The model under review builds one solid part; all positions refer to its coordinate system, in mm. A direction names the side the tool comes from. Coordinates: 2 decimals unless noted, no trailing zeros. Write each loop counter-clockwise with the first axis right and the second up, starting at its lowest first coordinate (ties: lowest second). Pieces come first, ordered by that corner, then holes. Notation, with made-up numbers: (51.5, 58.25) - (58.5, 58.25) arc R22 ccw to (58.5, 80.25) - close; hole circle Ø10 at (3, 83.25). An arc over 180 degrees is marked (long way). Use one line per item in the form item = value. Start each with the question number.
```python
from build123d import *

# Parameters (mm, degrees)
SKETCH1_W             = 18.7
SKETCH1_H             = 6.4
BOSS_EXTRUDE1_DEPTH   = 13
SKETCH2_W             = 13
SKETCH2_H             = 0.7
SKETCH2_W_2           = 0.5
SKETCH2_H_2           = 6.4
SKETCH2_W_3           = 1
BOSS_EXTRUDE2_DEPTH   = 2
CUT_EXTRUDE1_REACH    = 17
SKETCH3_R             = 0.9
CUT_EXTRUDE2_REACH    = 8.4
SKETCH5_R             = 1.1
CUT_EXTRUDE3_DEPTH    = 5.4
SKETCH6_R             = 1.1
CUT_EXTRUDE4_DEPTH    = 6.3
SKETCH7_R             = 1.1
CUT_EXTRUDE5_DEPTH    = 7
SKETCH8_R             = 1.1
CUT_EXTRUDE6_DEPTH    = 7.8
SKETCH10_W            = 6.4
SKETCH10_H            = 1
BOSS_EXTRUDE3_DEPTH   = 0.5
SKETCH11_W            = 6.4
SKETCH11_H            = 1
BOSS_EXTRUDE4_DEPTH   = 0.5
CHAMFER1_SIZE         = 0.5
CHAMFER1_SIZE2        = 0.3
CHAMFER1_PART_2_SIZE  = 0.5
CHAMFER1_PART_2_SIZE2 = 0.3


with BuildPart() as part:
    # Sketch1 → Boss-Extrude1 (new body)
    with BuildSketch(Plane(origin=(0, 0, 0), x_dir=(1, 0, 0), z_dir=(0, 1, 0))):
        Rectangle(SKETCH1_W, SKETCH1_H)
    extrude(amount=BOSS_EXTRUDE1_DEPTH)

    # Sketch2 → Boss-Extrude2 (add)
    with BuildSketch(Plane.XZ):
        with Locations((0.15, 2.85)):
            Rectangle(SKETCH2_W, SKETCH2_H)
        with Locations((0.15, -2.85)):
            Rectangle(SKETCH2_W, SKETCH2_H)
        with Locations((-9.1, 0)):
            Rectangle(SKETCH2_W_2, SKETCH2_H_2)
        with Locations((8.85, 0)):
            Rectangle(SKETCH2_W_3, SKETCH2_H_2)
    extrude(amount=BOSS_EXTRUDE2_DEPTH)

    # Sketch3 → Cut-Extrude1 (cut, up to next)
    with BuildSketch(Plane(origin=(0, 13, 0), x_dir=(1, 0, 0), z_dir=(0, 1, 0)), mode=Mode.PRIVATE) as cut_extrude1_sk1:
        with Locations(Location((4.25, -1.25, 0), (0, 0, 270))):  # turned: the seam where the file's is
            Circle(SKETCH3_R)
    cut_extrude1_tool1 = extrude(cut_extrude1_sk1.sketch, amount=-CUT_EXTRUDE1_REACH, mode=Mode.PRIVATE) & part.part
    add(cut_extrude1_tool1.solids().sort_by_distance((4.25, 13, 1.25))[0], mode=Mode.SUBTRACT)
    # Sketch3 → Cut-Extrude1 (cut, up to next)
    with BuildSketch(Plane(origin=(0, 13, 0), x_dir=(1, 0, 0), z_dir=(0, 1, 0)), mode=Mode.PRIVATE) as cut_extrude1_sk2:
        with Locations(Location((1.75, -1.25, 0), (0, 0, 270))):  # turned: the seam where the file's is
            Circle(SKETCH3_R)
    cut_extrude1_tool2 = extrude(cut_extrude1_sk2.sketch, amount=-CUT_EXTRUDE1_REACH, mode=Mode.PRIVATE) & part.part
    add(cut_extrude1_tool2.solids().sort_by_distance((1.75, 13, 1.25))[0], mode=Mode.SUBTRACT)
    # Sketch3 → Cut-Extrude1 (cut, up to next)
    with BuildSketch(Plane(origin=(0, 13, 0), x_dir=(1, 0, 0), z_dir=(0, 1, 0)), mode=Mode.PRIVATE) as cut_extrude1_sk3:
        with Locations(Location((-0.75, -1.25, 0), (0, 0, 270))):  # turned: the seam where the file's is
            Circle(SKETCH3_R)
    cut_extrude1_tool3 = extrude(cut_extrude1_sk3.sketch, amount=-CUT_EXTRUDE1_REACH, mode=Mode.PRIVATE) & part.part
    add(cut_extrude1_tool3.solids().sort_by_distance((-0.75, 13, 1.25))[0], mode=Mode.SUBTRACT)
    # Sketch3 → Cut-Extrude1 (cut, up to next)
    with BuildSketch(Plane(origin=(0, 13, 0), x_dir=(1, 0, 0), z_dir=(0, 1, 0)), mode=Mode.PRIVATE) as cut_extrude1_sk4:
        with Locations(Location((-3.25, -1.25, 0), (0, 0, 270))):  # turned: the seam where the file's is
            Circle(SKETCH3_R)
    cut_extrude1_tool4 = extrude(cut_extrude1_sk4.sketch, amount=-CUT_EXTRUDE1_REACH, mode=Mode.PRIVATE) & part.part
    add(cut_extrude1_tool4.solids().sort_by_distance((-3.25, 13, 1.25))[0], mode=Mode.SUBTRACT)
    # Sketch3 → Cut-Extrude1 (cut, up to next)
    with BuildSketch(Plane(origin=(0, 13, 0), x_dir=(1, 0, 0), z_dir=(0, 1, 0)), mode=Mode.PRIVATE) as cut_extrude1_sk5:
        with Locations(Location((4.25, 1.25, 0), (0, 0, 270))):  # turned: the seam where the file's is
            Circle(SKETCH3_R)
    cut_extrude1_tool5 = extrude(cut_extrude1_sk5.sketch, amount=-CUT_EXTRUDE1_REACH, mode=Mode.PRIVATE) & part.part
    add(cut_extrude1_tool5.solids().sort_by_distance((4.25, 13, -1.25))[0], mode=Mode.SUBTRACT)
    # Sketch3 → Cut-Extrude1 (cut, up to next)
    with BuildSketch(Plane(origin=(0, 13, 0), x_dir=(1, 0, 0), z_dir=(0, 1, 0)), mode=Mode.PRIVATE) as cut_extrude1_sk6:
        with Locations(Location((1.75, 1.25, 0), (0, 0, 270))):  # turned: the seam where the file's is
            Circle(SKETCH3_R)
    cut_extrude1_tool6 = extrude(cut_extrude1_sk6.sketch, amount=-CUT_EXTRUDE1_REACH, mode=Mode.PRIVATE) & part.part
    add(cut_extrude1_tool6.solids().sort_by_distance((1.75, 13, -1.25))[0], mode=Mode.SUBTRACT)
    # Sketch3 → Cut-Extrude1 (cut, up to next)
    with BuildSketch(Plane(origin=(0, 13, 0), x_dir=(1, 0, 0), z_dir=(0, 1, 0)), mode=Mode.PRIVATE) as cut_extrude1_sk7:
        with Locations(Location((-0.75, 1.25, 0), (0, 0, 270))):  # turned: the seam where the file's is
            Circle(SKETCH3_R)
    cut_extrude1_tool7 = extrude(cut_extrude1_sk7.sketch, amount=-CUT_EXTRUDE1_REACH, mode=Mode.PRIVATE) & part.part
    add(cut_extrude1_tool7.solids().sort_by_distance((-0.75, 13, -1.25))[0], mode=Mode.SUBTRACT)
    # Sketch3 → Cut-Extrude1 (cut, up to next)
    with BuildSketch(Plane(origin=(0, 13, 0), x_dir=(1, 0, 0), z_dir=(0, 1, 0)), mode=Mode.PRIVATE) as cut_extrude1_sk8:
        with Locations(Location((-3.25, 1.25, 0), (0, 0, 270))):  # turned: the seam where the file's is
            Circle(SKETCH3_R)
    cut_extrude1_tool8 = extrude(cut_extrude1_sk8.sketch, amount=-CUT_EXTRUDE1_REACH, mode=Mode.PRIVATE) & part.part
    add(cut_extrude1_tool8.solids().sort_by_distance((-3.25, 13, -1.25))[0], mode=Mode.SUBTRACT)

    # Sketch4 → Cut-Extrude2 (cut, up to next)
    with BuildSketch(Plane(origin=(0, 0, -3.2), x_dir=(-1, 0, 0), z_dir=(0, 0, -1)), mode=Mode.PRIVATE) as cut_extrude2_sk1:
        with BuildLine():
            Line((-9.35, 13), (9.35, 13))
            Line((9.35, 13), (9.35, 9.790050428))
            add(Edge.make_bspline(
                [(9.35, 9.790050428), (-0.455442008, 7.925691322), (-9.35, 3.892093752)],
                knots=[1.786761572, 1.786761572, 1.786761572, 2.052876958, 2.052876958, 2.052876958], degree=2, weights=[1, 0.991160878, 1]))
            Line((-9.35, 3.892093752), (-9.35, 13))
        make_face()
    cut_extrude2_tool1 = extrude(cut_extrude2_sk1.sketch, amount=-CUT_EXTRUDE2_REACH, mode=Mode.PRIVATE) & part.part
    add(cut_extrude2_tool1.solids().sort_by_distance((1.591729, 9.871634, -3.2))[0], mode=Mode.SUBTRACT)

    # Sketch5 → Cut-Extrude3 (cut)
    with BuildSketch(Plane.XZ):
        with Locations(Location((4.25, -1.25, 0), (0, 0, 270))):  # turned: the seam where the file's is
            Circle(SKETCH5_R)
        with Locations(Location((4.25, 1.25, 0), (0, 0, 270))):  # turned: the seam where the file's is
            Circle(SKETCH5_R)
    extrude(amount=-CUT_EXTRUDE3_DEPTH, mode=Mode.SUBTRACT)

    # Sketch6 → Cut-Extrude4 (cut)
    with BuildSketch(Plane.XZ):
        with Locations(Location((1.75, 1.25, 0), (0, 0, 270))):  # turned: the seam where the file's is
            Circle(SKETCH6_R)
        with Locations(Location((1.75, -1.25, 0), (0, 0, 270))):  # turned: the seam where the file's is
            Circle(SKETCH6_R)
    extrude(amount=-CUT_EXTRUDE4_DEPTH, mode=Mode.SUBTRACT)

    # Sketch7 → Cut-Extrude5 (cut)
    with BuildSketch(Plane.XZ):
        with Locations(Location((-0.75, 1.25, 0), (0, 0, 270))):  # turned: the seam where the file's is
            Circle(SKETCH7_R)
        with Locations(Location((-0.75, -1.25, 0), (0, 0, 270))):  # turned: the seam where the file's is
            Circle(SKETCH7_R)
    extrude(amount=-CUT_EXTRUDE5_DEPTH, mode=Mode.SUBTRACT)

    # Sketch8 → Cut-Extrude6 (cut)
    with BuildSketch(Plane.XZ):
        with Locations(Location((-3.25, 1.25, 0), (0, 0, 270))):  # turned: the seam where the file's is
            Circle(SKETCH8_R)
        with Locations(Location((-3.25, -1.25, 0), (0, 0, 270))):  # turned: the seam where the file's is
            Circle(SKETCH8_R)
    extrude(amount=-CUT_EXTRUDE6_DEPTH, mode=Mode.SUBTRACT)

    # Sketch10 → Boss-Extrude3 (add)
    with BuildSketch(Plane.ZY.offset(-8.35)):
        with Locations((0, -1.5)):
            Rectangle(SKETCH10_W, SKETCH10_H)
    extrude(amount=BOSS_EXTRUDE3_DEPTH)

    # Sketch11 → Boss-Extrude4 (add)
    with BuildSketch(Plane(origin=(-8.85, 0, 0), x_dir=(0, 0, -1), z_dir=(1, 0, 0))):
        with Locations((0, -1.5)):
            Rectangle(SKETCH11_W, SKETCH11_H)
    extrude(amount=BOSS_EXTRUDE4_DEPTH)

    # Chamfer1
    chamfer1_edges = [part.edges().sort_by_distance(p)[0] for p in [
        (7.85, -2, 0),
    ]]
    chamfer1_side = [part.faces().sort_by_distance(p)[0] for p in [
        (8.6, -2, 0),
    ]]
    chamfer(chamfer1_edges, length=CHAMFER1_SIZE, length2=CHAMFER1_SIZE2, reference=chamfer1_side[0])

    # Chamfer1 part 2
    chamfer1_part_2_edges = [part.edges().sort_by_distance(p)[0] for p in [
        (-8.35, -2, 0),
    ]]
    chamfer1_part_2_side = [part.faces().sort_by_distance(p)[0] for p in [
        (-8.85, -2, 0),
    ]]
    chamfer(chamfer1_part_2_edges, length=CHAMFER1_PART_2_SIZE, length2=CHAMFER1_PART_2_SIZE2, reference=chamfer1_part_2_side[0])


solid = part.part
```
1. For faces 3 (the cylindrical face through (-4.129, 8.129, 1.055)), 4 (the cylindrical face through (4.993, 2.662, -0.439)), list the 3-axis set-ups (+Z, -Z, +X, -X, +Y, -Y) from which the entire face can be reached by the end or side of a thin tool; tool diameter is ignored.
2. Take a section at A-A (y = -0.5). State the section outline as (x, z) points, plus the area to 3 significant figures.
3. Take a section at B-B (z = -1.25). Count the separate pieces of the cut face and the enclosed holes in it, plus the area to 3 significant figures.
4. The part is to be moulded in two halves that separate along Z. For faces 1 (the flat face through (-8.85, -0.5, 0)), 2 (the cylindrical face through (3.371, 5.767, 1.055)), say which applies: released by +Z, released by -Z, zero draft, split by the parting line, or undercut.
5. For L1, parallel to Z at x = -3.25, y = 8.1; L2, parallel to X at y = 3.25, z = 1.25; L3, parallel to Z at x = -3.75, y = 5.5, list the stretches that pass through material, from the lowest coordinate up.
6. For P1, Ø1.1, axis at x = 1.75, z = -1.25, coming from the +Y side; P2, Ø2, axis at x = 4.25, z = 1.25, coming from the -Y side; P3, Ø0.6, axis at x = -8.5, z = 0, coming from the +Y side; P4, Ø3, axis at x = -3, z = -0.5, coming from the +Y side, all flat-tipped, find the tip position at first contact; note any pin that passes through.
Returned:
q1.face_3 = +Y, -Y
q1.face_4 = -Y
q2.outline = (-9.35, -3.2) - (-8.85, -3.2) - (-8.85, 3.2) - (-9.35, 3.2) - close; (-6.35, -3.2) - (6.65, -3.2) - (6.65, -2.5) - (-6.35, -2.5) - close; (-6.35, 2.5) - (6.65, 2.5) - (6.65, 3.2) - (-6.35, 3.2) - close; (8.35, -3.2) - (9.35, -3.2) - (9.35, 3.2) - (8.35, 3.2) - close
q2.area = 27.8 mm²
q3.separate_pieces = 5
q3.enclosed_holes = 0
q3.area = 76.7 mm²
q4.face_1 = zero draft
q4.face_2 = undercut
q5.L1 = -3.2 to -2.15, -0.35 to 0.35, 2.15 to 3.2
q5.L2 = -9.35 to -4.35, -2.15 to -1.85, 0.35 to 0.65, 2.85 to 3.15, 5.35 to 9.35
q5.L3 = -3.2 to -2.23, -0.27 to 0.27, 2.23 to 3.2
q6.P1 = through
q6.P2 = 5.4
q6.P3 = 9.68
q6.P4 = 8.72
